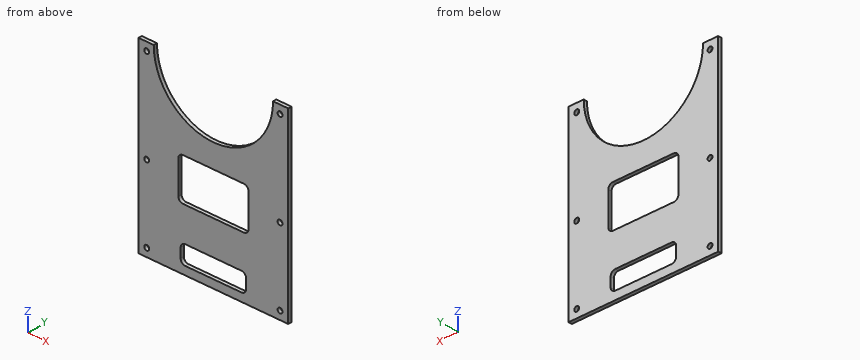
```python
from build123d import *

# Parameters (mm, degrees)
F1_DEPTH = 9.525
F2_R     = 6.6675
F3_DEPTH = 9.526


with BuildPart() as f1:
    # F0 (on Front) → F1 (new body)
    with BuildSketch(Plane.XZ):
        with BuildLine():
            ThreePointArc((161.925, 0), (0, -161.925), (-161.925, 0))
            Line((-161.925, 0), (-203.2, 0))
            Line((-203.2, 0), (-203.2, -504.825))
            Line((-203.2, -504.825), (203.2, -504.825))
            Line((203.2, -504.825), (203.2, 0))
            Line((203.2, 0), (161.925, 0))
        make_face()
        with BuildLine():
            Line((-88.9, -469.9), (-88.9, -444.5))
            ThreePointArc((-88.9, -444.5), (-85.180256, -435.519744), (-76.2, -431.8))
            Line((-76.2, -431.8), (76.2, -431.8))
            ThreePointArc((76.2, -431.8), (85.180256, -435.519744), (88.9, -444.5))
            Line((88.9, -444.5), (88.9, -469.9))
            ThreePointArc((88.9, -469.9), (85.180256, -478.880256), (76.2, -482.6))
            Line((76.2, -482.6), (-76.2, -482.6))
            ThreePointArc((-76.2, -482.6), (-85.180256, -478.880256), (-88.9, -469.9))
        make_face(mode=Mode.SUBTRACT)
        with BuildLine():
            Line((-95.25, -327.025), (-95.25, -238.125))
            ThreePointArc((-95.25, -238.125), (-91.530256, -229.144744), (-82.55, -225.425))
            Line((-82.55, -225.425), (82.55, -225.425))
            ThreePointArc((82.55, -225.425), (91.530256, -229.144744), (95.25, -238.125))
            Line((95.25, -238.125), (95.25, -327.025))
            ThreePointArc((95.25, -327.025), (91.530256, -336.005256), (82.55, -339.725))
            Line((82.55, -339.725), (-82.55, -339.725))
            ThreePointArc((-82.55, -339.725), (-91.530256, -336.005256), (-95.25, -327.025))
        make_face(mode=Mode.SUBTRACT)
    extrude(amount=F1_DEPTH)

    # F2 (on face) → F3 (cut, through all)
    with BuildSketch(Plane.XZ.offset(9.525)):
        with Locations((-180.975, -482.6)):
            Circle(F2_R)
        with Locations((180.975, -482.6)):
            Circle(F2_R)
        with Locations((-180.975, -22.225)):
            Circle(F2_R)
        with Locations((180.975, -22.225)):
            Circle(F2_R)
        with Locations((180.975, -276.225)):
            Circle(F2_R)
        with Locations((-180.975, -276.225)):
            Circle(F2_R)
    extrude(amount=-F3_DEPTH, mode=Mode.SUBTRACT)


solid = f1.part
```
Can you work these out from the model? Positions are in its coordinate system, mm. Give positions to 0.01 mm unless a question says otherwise; leave off trailing zeros. Order: outer loops, then holes, each group sorted by start corner. A loop starts at its lowest first (then second) coordinate and runs counter-clockwise, first axis right, second up. Notation, with made-up numbers: (22.5, -11) - (80.5, -11) arc R23 ccw to (80.5, 26) - close; hole circle Ø5 at (-25, 47). An arc over 180 degrees is marked (long way). Use a Markdown table: item, result. Add a question column.
Q1. If we section it at D-D on z = -132: Write out the boundary of the cut face in (x, y) (3 decimals).
Q2. I'm going to push a flat-ended pin straight in: pin 1 (3 mm diameter, centred on x = -4, y = -5.5, fed in from +Z). Where does the tip first touch, or does it pass through?
Q3. If we section it at B-B on z = -249: Write out the boundary of the cut face in (x, y) (3 decimals).
Q4. Please list where these lines run through material, in increasing order: line 1 along Z through (x, y) = (70.5, -6.75) (3 decimals); line 2 along X through (y, z) = (-2.5, -289); line 3 along Z through (x, y) = (-63, -6.5) (3 decimals).
Q5. If we section it at A-A on x = 0: Write out the boundary of the cut face in (y, z) (3 decimals).
Q6. If we section it at C-C on y = -7.25: Count the separate pieces of the cut face and the enclosed holes in it, plus the area to 3 significant figures.
Answers follow:
| question | item | result |
|---|---|---|
| 1 | outline | (-203.2, -9.525) - (-93.785, -9.525) - (-93.785, 0) - (-203.2, 0) - close; (93.785, -9.525) - (203.2, -9.525) - (203.2, 0) - (93.785, 0) - close |
| 2 | pin 1 | stops at z = -161.83 |
| 3 | outline | (-203.2, -9.525) - (-95.25, -9.525) - (-95.25, 0) - (-203.2, 0) - close; (95.25, -9.525) - (203.2, -9.525) - (203.2, 0) - (95.25, 0) - close |
| 4 | line 1 | z = -504.825 to -482.6, -431.8 to -339.725, -225.425 to -145.772 |
| 4 | line 2 | x = -203.2 to -95.25, 95.25 to 203.2 |
| 4 | line 3 | z = -504.825 to -482.6, -431.8 to -339.725, -225.425 to -149.167 |
| 5 | outline | (-9.525, -504.825) - (0, -504.825) - (0, -482.6) - (-9.525, -482.6) - close; (-9.525, -431.8) - (0, -431.8) - (0, -339.725) - (-9.525, -339.725) - close; (-9.525, -225.425) - (0, -225.425) - (0, -161.925) - (-9.525, -161.925) - close |
| 6 | separate pieces | 1 |
| 6 | enclosed holes | 8 |
| 6 | area | 133,000 mm^2 |
